The listing builds one solid part. Answer for the finished solid, in the listing's coordinates (mm). Face numbers are marked on the shaded views. A direction names the side the tool comes from. Give positions to 0.01 mm unless a question says otherwise; leave off trailing zeros. Loops run counter-clockwise (first coordinate to the right, second up) from the corner with the lowest first, then second, coordinate; pieces in that order, holes last. Notation, with made-up numbers: (82, 30) - (90, 30) arc R25 ccw to (90, 65) - close; hole circle Ø5 at (-21, 9). An arc over 180 degrees is marked (long way). Answer as CSV lines item,"result". Start each with the question number.
1) Find the intervals of material crossed by line 1 along Z through (x, y) = (30.5, 0); line 2 along X through (y, z) = (-3, 0); line 3 along Z through (x, y) = (67, 0), in increasing order.
2) For a pull along Z with two mould halves and no side action, classify the marked faces 6, 7, 8 and 9 as pulls with the +Z half, pulls with the -Z half, needs draft (parallel to the pull), parting line crosses it, or undercut.
3) A cutting plane is placed at A-A (x = 23.5). Determine the outline of the cut face in (y, z), and give its area (3 significant figures).
4) For the marked faces 1, 2, 3, 4 and 5, determine the directions among +Z, -Z, +X, -X, +Y, -Y from which every point of the face is accessible in a straight line to the end or side of a thin tool.
5) Flat-ended cylindrical pins translate along their axes: pin 1 (18.5 mm diameter, centred on x = 11.5, z = -24, fed in from -Y); pin 2 (18.5 mm diameter, centred on x = 10, z = 31.5, fed in from +Y); pin 3 (11.5 mm diameter, centred on x = 67.5, z = 0, fed in from +Y). Find the tip coordinate at first contact, or state that the pin passes through.
6) A cutting plane is placed at C-C (z = 37). Determine the outline of the cut face in (x, y), and give its area (3 significant figures).
7) A cutting plane is placed at B-B (x = 47). Determine the outline of the cut face in (y, z).
8) A cutting plane is placed at D-D (y = 32). Determine the outline of the cut face in (x, z).
```python
from build123d import *

# Parameters (mm, degrees)
SKETCH_2_R          = 20
EXTRUDE_1_DEPTH     = 50
CUT_EXTRUDE_2_DEPTH = 30
CUT_EXTRUDE_3_DEPTH = 30
SKETCH_5_W          = 55
SKETCH_5_H          = 45
EXTRUDE_2_DEPTH     = 45
FILLET_2_R          = 27.5
FILLET_3_R          = 27.5
CHAMFER_1_SIZE      = 5
SKETCH_6_R          = 5
CUT_EXTRUDE_4_DEPTH = 123.737864302
CHAMFER_2_SIZE      = 5


with BuildPart() as part:
    # 스케치2 → 보스-돌출1 (new body)
    with BuildSketch(Plane(origin=(0, 0, 0), x_dir=(0, 0, -1), z_dir=(1, 0, 0))):
        Polygon((46.188021535, 0), (23.094010768, 40), (-23.094010768, 40), (-46.188021535, 0), (-23.094010768, -40), (23.094010768, -40), align=None)
        Circle(SKETCH_2_R, mode=Mode.SUBTRACT)
    extrude(amount=EXTRUDE_1_DEPTH)

    # 스케치3 → 컷-돌출2 (cut)
    with BuildSketch(Plane.ZY):
        with BuildLine():
            ThreePointArc((-17.320508076, 10), (0, 20), (17.320508076, 10))
            Line((17.320508076, 10), (40.414518843, 10))
            Line((40.414518843, 10), (23.094010768, 40))
            Line((23.094010768, 40), (-23.094010768, 40))
            Line((-23.094010768, 40), (-40.414518843, 10))
            Line((-40.414518843, 10), (-17.320508076, 10))
        make_face()
    extrude(amount=-CUT_EXTRUDE_2_DEPTH, mode=Mode.SUBTRACT)

    # 스케치3<4> → 컷-돌출3 (cut)
    with BuildSketch(Plane.ZY):
        with BuildLine():
            Line((40.414518843, -10), (17.320508076, -10))
            ThreePointArc((17.320508076, -10), (0, -20), (-17.320508076, -10))
            Line((-17.320508076, -10), (-40.414518843, -10))
            Line((-40.414518843, -10), (-23.094010768, -40))
            Line((-23.094010768, -40), (23.094010768, -40))
            Line((23.094010768, -40), (40.414518843, -10))
        make_face()
    extrude(amount=-CUT_EXTRUDE_3_DEPTH, mode=Mode.SUBTRACT)

    # 스케치5 → 보스-돌출2 (add)
    with BuildSketch(Plane(origin=(50, 0, 0), x_dir=(0, 0, -1), z_dir=(1, 0, 0))):
        Rectangle(SKETCH_5_W, SKETCH_5_H)
    extrude(amount=EXTRUDE_2_DEPTH)

    # 필렛2
    fillet_2_edges = [part.edges().sort_by_distance(p)[0] for p in [
        (95, 0, -27.5),
    ]]
    fillet(fillet_2_edges, radius=FILLET_2_R)

    # 필렛3
    fillet_3_edges = [part.edges().sort_by_distance(p)[0] for p in [
        (95, 0, 27.5),
    ]]
    fillet(fillet_3_edges, radius=FILLET_3_R - 0.0001)  # a hair under: the kernel refuses the full size

    # 모따기1
    chamfer_1_edges = [part.edges().sort_by_distance(p)[0] for p in [
        (58.75, -22.5, -27.5),
        (86.945436483, -22.5, -19.445436483),
        (58.75005, -22.5, 27.5),
        (86.945465772, -22.5, 19.445465772),
    ]]
    chamfer(chamfer_1_edges, length=CHAMFER_1_SIZE)

    # 스케치6 → 컷-돌출4 (cut, through all)
    with BuildSketch(Plane.XZ.offset(22.5)):
        with Locations(Location((67.5, 0, 0), (0, 0, 270))):
            Circle(SKETCH_6_R)
    extrude(amount=-CUT_EXTRUDE_4_DEPTH, mode=Mode.SUBTRACT)

    # 모따기2
    chamfer_2_edges = [part.edges().sort_by_distance(p)[0] for p in [
        (58.75, 22.5, -27.5),
        (86.945436483, 22.5, -19.445436483),
        (58.75005, 22.5, 27.5),
        (86.945465772, 22.5, 19.445465772),
    ]]
    chamfer(chamfer_2_edges, length=CHAMFER_2_SIZE)


solid = part.part
```
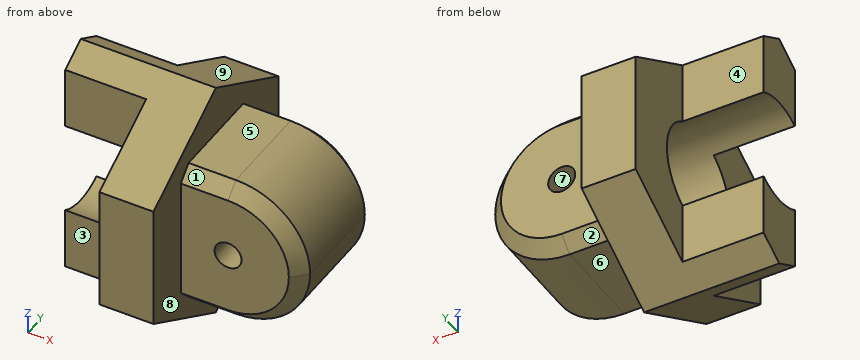
Ans:
1,line 1,"-46.19 to -20, 20 to 46.19"
1,line 2,"50 to 62.5, 72.5 to 95"
1,line 3,"-27.5 to -4.97, 4.97 to 27.5"
2,face 6,"pulls with the -Z half"
2,face 7,"undercut"
2,face 8,"needs draft"
2,face 9,"pulls with the +Z half"
3,outline,"(-10, -40.41) - (0, -46.19) - (10, -40.41) - (10, -17.32) arc R20 cw to (-10, -17.32) - close; (-10, 17.32) arc R20 cw to (10, 17.32) - (10, 40.41) - (0, 46.19) - (-10, 40.41) - close"
3,area,"967 mm2"
4,face 1,"+Z, +X, -Y"
4,face 2,"-Z, +X, +Y"
4,face 3,"+Z, -Z, -X, -Y"
4,face 4,"+Z, -Z, -X, +Y"
4,face 5,"+Z, +X, +Y, -Y"
5,pin 1,"y = -10"
5,pin 2,"y = 10"
5,pin 3,"y = 22.5"
6,outline,"(0, -10) - (30, -10) - (30, -15.91) - (50, -15.91) - (50, 15.91) - (30, 15.91) - (30, 10) - (0, 10) - close"
6,area,"1,240 mm2"
7,outline,"(-40, -23.09) - (0, -46.19) - (40, -23.09) - (40, 23.09) - (0, 46.19) - (-40, 23.09) - close; hole circle Ø40 at (0, 0)"
8,outline,"(30, -27.71) - (50, -27.71) - (50, 27.71) - (30, 27.71) - close"
